The listing builds one solid part. Answer for the finished solid, in the listing's coordinates (mm). Face numbers are marked on the shaded views. Coordinates: 2 decimals unless noted, no trailing zeros. Write each loop counter-clockwise with the first axis right and the second up, starting at its lowest first coordinate (ties: lowest second). Pieces come first, ordered by that corner, then holes.
(1) The part is cut by section A-A on x = 64. Determine the outline of the cut face in (y, z).
(2) For a pull along Y with two mould halves and no side action, classify the marked faces 1, 2, 3 and 4 as +Y half, -Y half, draft (parallel to the pull), parting line (faces both ways), or undercut.
(3) Straight lines are drawn through the part: line 1 (X direction, y = -51, z = 0); line 2 (Z direction, x = 75.1, y = -47.75); line 3 (Y direction, x = 33, z = -4). For each, find the intervals that lie inside material, in ascending order.
(4) The part is cut by section C-C on x = 33.5. Determine the outline of the cut face in (y, z).
(5) The part is cut by section B-B on y = -22. Determine the outline of the cut face in (x, z), plus the area to 3 significant figures.
(6) Given P1, Ø4, axis at x = -42.5, z = 0, coming from the +Y side; P2, Ø6, axis at x = 16.3, z = 0, coming from the +Y side, each flat-ended and moving along its own axis, determine where each tip first touches the part or whether it passes through.
(7) The part is cut by section D-D on y = 25. Determine the outline of the cut face in (x, z).
from build123d import *

# Parameters (mm, degrees)
CROQUIS1_R                = 45
SALIENTE_EXTRUIR1_DEPTH   = 7.5
TALADRO_ROSCADO_M81_D     = 6.8
TALADRO_ROSCADO_M81_DEPTH = 20
TALADRO_ROSCADO_M81_TIP   = 2.042926105
TALADRO_ROSCADO_M82_D     = 6.8
TALADRO_ROSCADO_M82_DEPTH = 10
TALADRO_ROSCADO_M82_TIP   = 2.042926105
CORTAR_EXTRUIR1_DEPTH     = 167.9


with BuildPart() as part:
    # Croquis1 → Saliente-Extruir1 (new body, symmetric)
    with BuildSketch(Plane.XY):
        with BuildLine():
            Line((-50, -55), (-50, 59.973896209))
            ThreePointArc((-50, 59.973896209), (-45.047974372, 71.111140529), (-33.461571863, 74.894795608))
            Line((-33.461571863, 74.894795608), (111, 60))
            Line((111, 60), (111, -55))
            Line((111, -55), (-50, -55))
        make_face()
        Circle(CROQUIS1_R, mode=Mode.SUBTRACT)
        with BuildLine():
            ThreePointArc((65.982119452, -11.634427904), (47.376154339, 47.376154339), (-11.634427904, 65.982119452))
            ThreePointArc((-11.634427904, 65.982119452), (-14.879066205, 61.348295729), (-10.245242482, 58.103657428))
            ThreePointArc((-10.245242482, 58.103657428), (41.71930009, 41.71930009), (58.103657428, -10.245242482))
            ThreePointArc((58.103657428, -10.245242482), (61.348295729, -14.879066205), (65.982119452, -11.634427904))
        make_face(mode=Mode.SUBTRACT)
    extrude(amount=SALIENTE_EXTRUIR1_DEPTH, both=True)

    # Taladro roscado M81
    with Locations(Plane(origin=(111, 0, 0), x_dir=(0, 0, -1), z_dir=(1, 0, 0))):
        with Locations((0, 52.5), (0, 2.5), (0, -47.5)):
            Hole(TALADRO_ROSCADO_M81_D / 2, depth=TALADRO_ROSCADO_M81_DEPTH)
            with Locations((0, 0, -(TALADRO_ROSCADO_M81_DEPTH + TALADRO_ROSCADO_M81_TIP / 2))):  # 118° drill point
                Cone(0, TALADRO_ROSCADO_M81_D / 2, TALADRO_ROSCADO_M81_TIP, mode=Mode.SUBTRACT)

    # Taladro roscado M82
    with Locations(Plane.XZ.offset(55)):
        with Locations((-42.5, 0), (16.3, 0), (75.1, 0)):
            Hole(TALADRO_ROSCADO_M82_D / 2, depth=TALADRO_ROSCADO_M82_DEPTH)
            with Locations((0, 0, -(TALADRO_ROSCADO_M82_DEPTH + TALADRO_ROSCADO_M82_TIP / 2))):  # 118° drill point
                Cone(0, TALADRO_ROSCADO_M82_D / 2, TALADRO_ROSCADO_M82_TIP, mode=Mode.SUBTRACT)

    # Croquis7 → Cortar-Extruir1 (cut)
    with BuildSketch(Plane.XZ.offset(55)):
        Polygon((-50, 7.5), (-50, 3.5), (-46, 7.5), align=None)
        Polygon((-50, -7.5), (-50, -3.5), (-46, -7.5), align=None)
    extrude(amount=-CORTAR_EXTRUIR1_DEPTH, mode=Mode.SUBTRACT)


solid = part.part
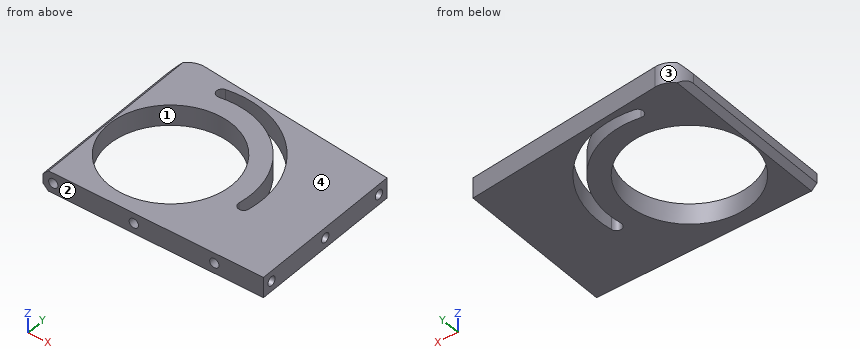
Model answer:
1. outline: (-55, -7.5) - (-14.43, -7.5) - (-14.43, 7.5) - (-55, 7.5) - close; (19.82, -7.5) - (64.85, -7.5) - (64.85, 7.5) - (19.82, 7.5) - close
2. face 1: undercut
2. face 2: -Y half
2. face 3: +Y half
2. face 4: draft
3. line 1: x = -50 to -45.9, -39.1 to 12.9, 19.7 to 71.7, 78.5 to 111
3. line 2: z = -7.5 to -3.4, 3.4 to 7.5
3. line 3: y = -55 to -30.59, 30.59 to 48.91, 58.31 to 68.04
4. outline: (-55, -7.5) - (-30.05, -7.5) - (-30.05, 7.5) - (-55, 7.5) - close; (30.05, -7.5) - (48.57, -7.5) - (48.57, 7.5) - (30.05, 7.5) - close; (58.02, -7.5) - (67.99, -7.5) - (67.99, 7.5) - (58.02, 7.5) - close
5. outline: (-50, -3.5) - (-46, -7.5) - (-39.26, -7.5) - (-39.26, 7.5) - (-46, 7.5) - (-50, 3.5) - close; (39.26, -7.5) - (111, -7.5) - (111, 7.5) - (39.26, 7.5) - close
5. area: 1,220 mm2
6. P1: stops at y = 73.93
6. P2: stops at y = 70.07
7. outline: (-50, -3.5) - (-46, -7.5) - (-37.42, -7.5) - (-37.42, 7.5) - (-46, 7.5) - (-50, 3.5) - close; (37.42, -7.5) - (53.44, -7.5) - (53.44, 7.5) - (37.42, 7.5) - close; (62.16, -7.5) - (111, -7.5) - (111, 7.5) - (62.16, 7.5) - close
